Source: CAD feature listing. Evaluate the final solid. Frame: model axes, mm. Coordinates: 2 decimals unless noted, no trailing zeros. Order: outer loops, then holes, each group sorted by start corner. A loop starts at its lowest first (then second) coordinate and runs counter-clockwise, first axis right, second up.
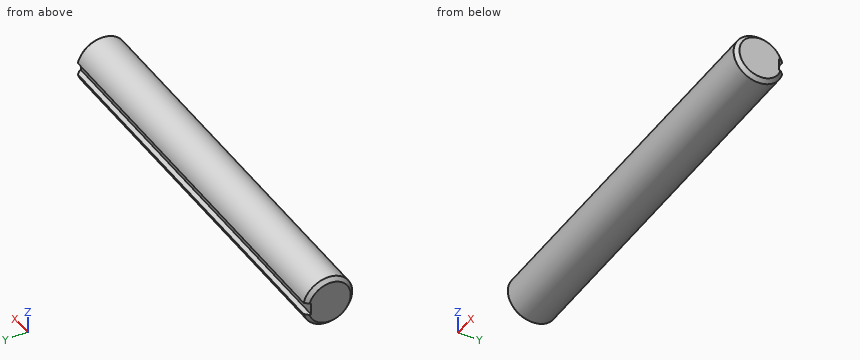
```python
from build123d import *

# Parameters (mm, degrees)
SKETCH1_R           = 19.05
EXTRUDE1_DEPTH      = 152.4
CHAMFER1_SIZE       = 2.8575
SKETCH3_W           = 9.525
SKETCH3_H           = 4.7625
EXTRUDE2_DEPTH      = 153.4
EXTRUDE2_DEPTH_BACK = 153.4


with BuildPart() as part:
    # Sketch1 → Extrude1 (new body, symmetric)
    with BuildSketch(Plane(origin=(0, 0, 0), x_dir=(0, 0, -1), z_dir=(1, 0, 0))):
        Circle(SKETCH1_R)
    extrude(amount=EXTRUDE1_DEPTH, both=True)

    # Chamfer1
    chamfer1_edges = [part.edges().sort_by_distance(p)[0] for p in [
        (-152.4, 0, 19.05),
        (152.4, 0, 19.05),
    ]]
    chamfer(chamfer1_edges, length=CHAMFER1_SIZE)

    # Sketch3 → Extrude2 (cut, two sides)
    with BuildSketch(Plane.ZY) as extrude2_sk:
        with Locations((0, 16.66875)):
            Rectangle(SKETCH3_W, SKETCH3_H)
    extrude(amount=EXTRUDE2_DEPTH, mode=Mode.SUBTRACT)
    extrude(extrude2_sk.sketch, amount=-EXTRUDE2_DEPTH_BACK, mode=Mode.SUBTRACT)


solid = part.part
```
1. Section query B-B on x = -46. Return loops of the section in (y, z).
Findings:
outline: (14.29, -4.76) - (14.29, 4.76) - (18.45, 4.76) arc R19.05 ccw (long way) to (18.45, -4.76) - close
2. Section query A-A on z = 0. Return loops of the section in (x, y).
Findings:
outline: (-152.4, -16.19) - (-149.54, -19.05) - (149.54, -19.05) - (152.4, -16.19) - (152.4, 14.29) - (-152.4, 14.29) - close
3. Pin query (flat end, axial travel): P1, Ø3, axis at x = 49, z = 2, coming from the +Y side; P2, Ø10, axis at x = 72, z = -1.5, coming from the -Y side; P3, Ø4.5, axis at x = 19.5, y = 16, coming from the +Z side. Return the tip coordinate at first contact, or that it passes through.
Findings:
P1: stops at y = 14.29
P2: stops at y = -19.05
P3: stops at z = 13.18
4. Ray query, line 1 (Y direction, x = 73, z = 0.5); line 2 (Z direction, x = 63, y = 17); line 3 (Z direction, x = -94.5, y = 14.5). Return the intervals inside material, ascending.
Findings:
line 1: y = -19.04 to 14.29
line 2: z = -8.6 to -4.76, 4.76 to 8.6
line 3: z = -12.36 to -4.76, 4.76 to 12.36
